Read the model definition and answer for the solid it produces. Units are mm, in the model's axes. Round coordinates to 2 decimals unless told otherwise and drop trailing zeros. Write each loop counter-clockwise with the first axis right and the second up, starting at its lowest first coordinate (ties: lowest second). Pieces come first, ordered by that corner, then holes.
from build123d import *

# Parameters (mm, degrees)
SKETCH1_W                        = 19.05
SKETCH1_H                        = 96.52
BOSS_EXTRUDE1_DEPTH              = 12.7
F_3_8_16_TAPPED_HOLE1_AT_2_COUNT = 2
F_3_8_16_TAPPED_HOLE1_AT_2_PITCH = 76.2
CHAMFER1_SIZE                    = 1.524


with BuildPart() as part:
    # Sketch1 → Boss-Extrude1 (new body)
    with BuildSketch(Plane.XY):
        Rectangle(SKETCH1_W, SKETCH1_H)
    extrude(amount=-BOSS_EXTRUDE1_DEPTH)

    # Sketch18 → 3/8-16 Tapped Hole1 (revolve, cut)
    with BuildSketch(Plane(origin=(0, -38.1, 0), x_dir=(0, -1, 0), z_dir=(1, 0, 0))):
        Polygon((0, 0), (0, 29.384865582), (3.96875, 27.0002), (3.96875, 19.05), (4.7625, 19.05), (4.7625, 0.635), (5.3975, 0), align=None)
    f_3_8_16_tapped_hole1 = revolve(axis=Axis((0, -38.1, 6.35), (0, 0, -1)), mode=Mode.SUBTRACT)

    # 3/8-16 Tapped Hole1 at 2: 3/8-16 Tapped Hole1 ×2
    with Locations(*[(0, i * F_3_8_16_TAPPED_HOLE1_AT_2_PITCH, 0) for i in range(1, F_3_8_16_TAPPED_HOLE1_AT_2_COUNT)]):
        add(f_3_8_16_tapped_hole1, mode=Mode.SUBTRACT)

    # Chamfer1
    chamfer1_edges = [part.edges().sort_by_distance(p)[0] for p in [
        (-9.525, 48.26, -6.35),
        (9.525, 48.26, -6.35),
        (9.525, -48.26, -6.35),
        (-9.525, -48.26, -6.35),
    ]]
    chamfer(chamfer1_edges, length=CHAMFER1_SIZE)


solid = part.part
Q1. Determine the mould class of faces 1 (the flat face through (0, 1, -12.7)), 2 (the flat face through (0, 1, 0)), 3 (the cylindrical face through (-0.209, 42.858, -6.583)) for opening direction Z: pulls with the +Z half, pulls with the -Z half, needs draft (parallel to the pull), parting line crosses it, or undercut.
Verdict:
face 1: pulls with the -Z half
face 2: pulls with the +Z half
face 3: needs draft
Q2. Section D-D (x = 3.75) is taken. State how many separate pieces and enclosed holes the cut face has, then the cut area to 3 significant figures.
Verdict:
separate pieces: 3
enclosed holes: 0
area: 1,080 mm2
Q3. Section A-A (y = 38.1) is taken. Determine the outline of the cut face in (x, z) (1 decimal), then the cut area to 3 significant figures.
Verdict:
outline: (-9.5, -12.7) - (-4.8, -12.7) - (-4.8, -0.6) - (-5.4, 0) - (-9.5, 0) - close; (4.8, -12.7) - (9.5, -12.7) - (9.5, 0) - (5.4, 0) - (4.8, -0.6) - close
area: 121 mm2
Q4. Straight lines are drawn through the part: probe 1 along Y at (x, z) = (0, -7.25); probe 2 along X at (y, z) = (-38.1, -4.75) (1 decimal); probe 3 along Y at (x, z) = (-2.5, -10.25). For each, find the intervals that lie inside material, in ascending order.
Verdict:
probe 1: y = -48.26 to -42.86, -33.34 to 33.34, 42.86 to 48.26
probe 2: x = -9.5 to -4.8, 4.8 to 9.5
probe 3: y = -48.26 to -42.15, -34.05 to 34.05, 42.15 to 48.26
Q5. A flat-ended cylindrical pin translates along its axis: pin 1 Ø6 at (x, y) = (0.5, -15) entering from +Z. Find the tip coordinate at first contact, or state that the pin passes through.
Verdict:
pin 1: stops at z = 0
Q6. Section B-B (x = 0) is taken. Determine the outline of the cut face in (y, z) (1 decimal).
Verdict:
outline: (-48.3, -12.7) - (-42.9, -12.7) - (-42.9, -0.6) - (-43.5, 0) - (-48.3, 0) - close; (-33.3, -12.7) - (33.3, -12.7) - (33.3, -0.6) - (32.7, 0) - (-32.7, 0) - (-33.3, -0.6) - close; (42.9, -12.7) - (48.3, -12.7) - (48.3, 0) - (43.5, 0) - (42.9, -0.6) - close
Q7. Section C-C (z = -3.25) is taken. Determine the outline of the cut face in (x, y) (1 decimal), then the cut area to 3 significant figures.
Verdict:
outline: (-9.5, -46.7) - (-8, -48.3) - (8, -48.3) - (9.5, -46.7) - (9.5, 46.7) - (8, 48.3) - (-8, 48.3) - (-9.5, 46.7) - close; hole circle Ø9.5 at (0, -38.1); hole circle Ø9.5 at (0, 38.1)
area: 1,690 mm2
